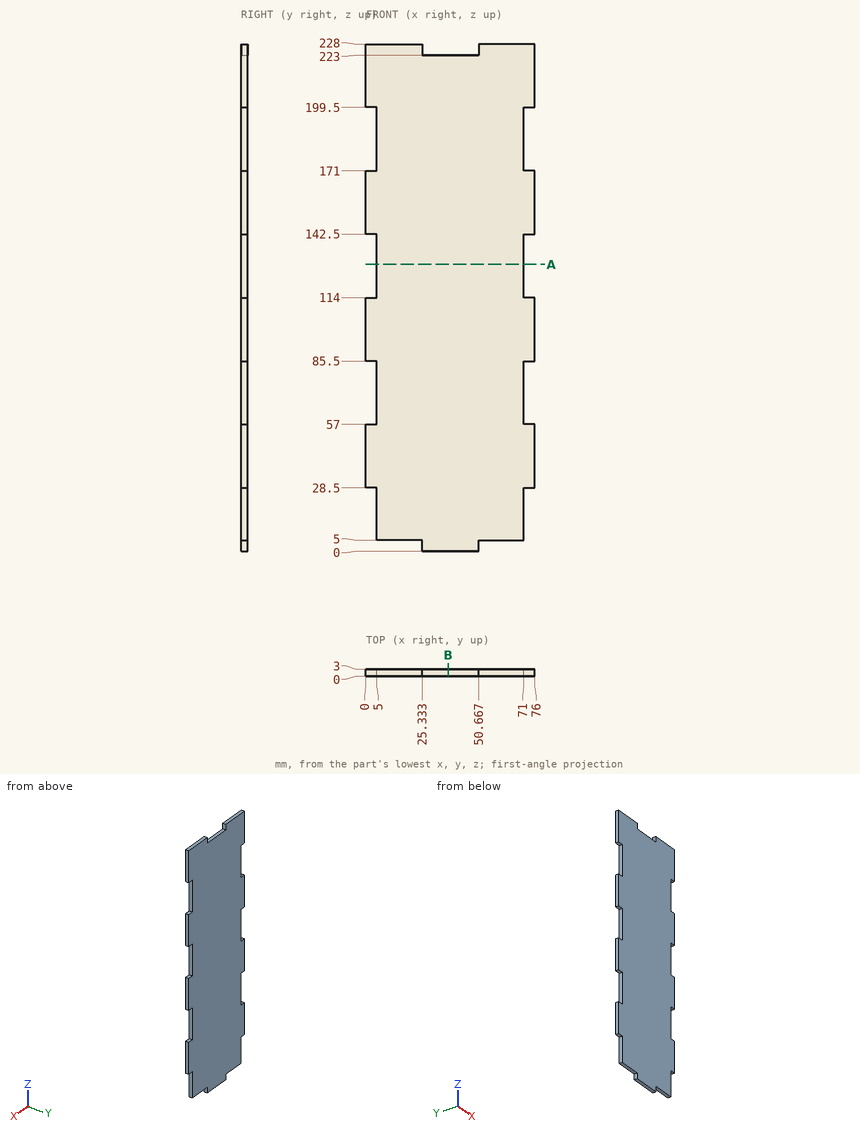
Can you work these out from the drawing? Everything is in mm from the part's minimum corner. Coordinates: 2 decimals unless noted, no trailing zeros. Write each loop counter-clockwise with the first axis right and the second up, starting at its lowest first coordinate (ties: lowest second). Pieces come first, ordered by that corner, then holes. Notation, with made-up numbers: (37.25, 51) -> (94.25, 51) arc R24 ccw to (94.25, 89) -> close; hole circle Ø2 at (58, 24). An arc over 180 degrees is marked (long way). Write each question's results on one line, items separated by ' | '. Start each with the question number.
Q1. If I drill on probe 1 along X at (y, z) = (1, 77.5); probe 2 along Z at (x, y) = (39, 1.45); probe 3 along Z at (x, y) = (21, 1.4), over which ranges is the centre line in solid material (lowest first)?
Q2. Imagine slicing it at B-B (x = 37). Write out the boundary of the cut face in (y, z).
Q3. I'm going to push flat-ended pins straight in: pin 1 (1.5 mm diameter, centred on x = 29.5, y = 2.5, fed in from -Z); pin 2 (0.9 mm diameter, centred on y = 1, z = 189, fed in from -X); pin 3 (1.5 mm diameter, centred on x = 58.5, y = 1.5, fed in from -Z); pin 4 (0.9 mm diameter, centred on x = 1.5, y = 2, fed in from -Z). Where does each tip first touch, or does it pass through?
Q4. Imagine slicing it at A-A (z = 129). Write out the boundary of the cut face in (x, y), then the cut area to 3 significant figures.
Taken from the geometry:
1) probe 1: x = 5 to 71 | probe 2: z = 0 to 223 | probe 3: z = 5 to 228
2) outline: (0, 0) -> (3, 0) -> (3, 223) -> (0, 223) -> close
3) pin 1: stops at z = 0 | pin 2: stops at x = 5 | pin 3: stops at z = 5 | pin 4: stops at z = 28.5
4) outline: (5, 0) -> (71, 0) -> (71, 3) -> (5, 3) -> close | area: 198 mm^2
